For this review, take the finished solid that the model builds, in its own axes (mm). Face numbers are marked on the shaded views. Coordinates: 2 decimals unless noted, no trailing zeros. Order: outer loops, then holes, each group sorted by start corner. A loop starts at its lowest first (then second) coordinate and runs counter-clockwise, first axis right, second up. Notation, with made-up numbers: (-14.5, 51) -> (23.5, 51) arc R13 ccw to (23.5, 70) -> close; hole circle Ø9 at (-21, 27.5). An arc over 180 degrees is marked (long way). Answer as a JSON object with one key per item and string values. Group by question number.
1) For pin 1 (1 mm diameter, centred on x = -3, z = -14.5, fed in from -Y); pin 2 (3 mm diameter, centred on x = -4, z = -4, fed in from +Y); pin 3 (1 mm diameter, centred on x = -7, y = 4, fed in from -Z), all flat-tipped, find the tip position at first contact; note any pin that passes through.
2) Add section C-C, the plane z = -4.5. Write out the cut boundary in (x, y).
3) Draft analysis for pull direction Z (two halves, no side actions). For the marked faces 1, 2 and 3, state which applies: +Z half, -Z half, draft (parallel to the pull), parting line (faces both ways), or undercut.
4) Add section D-D, the plane x = -7. Write out the cut boundary in (y, z).
5) Add section A-A, the plane x = -4.5. Write out the cut boundary in (y, z).
6) Add section B-B, the plane y = 1.25. Count the separate pieces of the cut face and the enclosed holes in it, then the cut area to 3 significant figures.
7) Wall thickness on L1, parallel to Z at x = -4, y = 1.7; L2, parallel to X at y = 3.95, z = -4; L3, parallel to Z at x = -5.75, y = 3.4: over which ranges is each line inside the solid? List them lowest first.
Autodesk Inventor part; units mm, degrees
ref_plane "YZ Plane" through (0, 0, 0) normal (1, 0, 0) x (0, 1, 0)
ref_plane "XZ Plane" through (0, 0, 0) normal (0, 1, 0) x (-1, 0, 0)
ref_plane "XY Plane" through (0, 0, 0) normal (0, 0, 1) x (1, 0, 0)
sketch "Sketch1" plane through (0, 0, 0) normal (0, 1, 0) x (-1, 0, 0)
  line L0 (0, 0) -> (8, 0)
  line L1 (8, 0) -> (8, -45)
  line L2 (8, -45) -> (0, -45)
  line L3 (0, -45) -> (0, 0)
  line L4 (8, 0) -> (4, 0)
  line L5 (4, 0) -> (4, -4)
  circle A0 centre (4, -4) radius 2
  line L6 (8, -45) -> (4, -45)
  line L7 (4, -45) -> (4, -41)
  circle A1 centre (4, -41) radius 2
  dimension "d0" = 8
  dimension "d1" = 45
  dimension "d2" = 4
  dimension "d3" = 4
  dimension "d4" = 4
  dimension "d5" = 4
  dimension "d6" = 4
  dimension "d7" = 4
extrude "Extrusion1" add sketch "Sketch1" along normal blind 5
fillet "Fillet1" radius 4 4 edges at (0, 2.5, 0) (-8, 2.5, 0) (-8, 2.5, -45) (0, 2.5, -45)
properties part number "Bar"
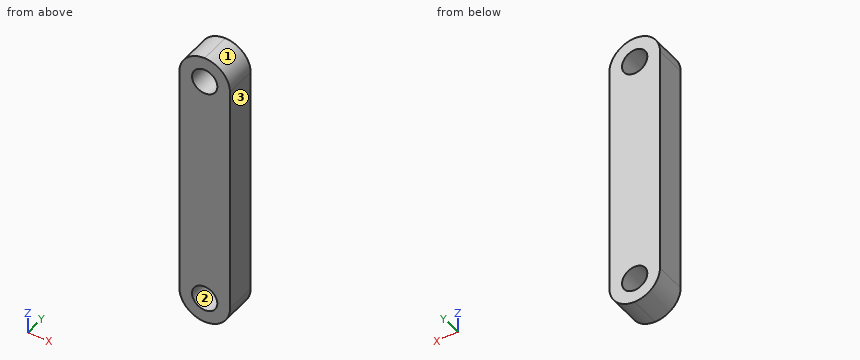
Output values:
{
 "1": {"pin 1": "stops at y = 0", "pin 2": "passes through", "pin 3": "stops at z = -44.12"},
 "2": {"outline": "(-8, 0) -> (-5.94, 0) -> (-5.94, 5) -> (-8, 5) -> close; (-2.06, 0) -> (0, 0) -> (0, 5) -> (-2.06, 5) -> close"},
 "3": {"face 1": "+Z half", "face 2": "undercut", "face 3": "draft"},
 "4": {"outline": "(0, -43.65) -> (5, -43.65) -> (5, -1.35) -> (0, -1.35) -> close"},
 "5": {"outline": "(0, -44.97) -> (5, -44.97) -> (5, -42.94) -> (0, -42.94) -> close; (0, -39.06) -> (5, -39.06) -> (5, -5.94) -> (0, -5.94) -> close; (0, -2.06) -> (5, -2.06) -> (5, -0.03) -> (0, -0.03) -> close"},
 "6": {"separate pieces": "1", "enclosed holes": "2", "area": "321 mm²"},
 "7": {"L1": "z = -45 to -43, -39 to -6, -2 to 0", "L2": "x = -8 to -6, -2 to 0", "L3": "z = -44.6 to -41.97, -40.03 to -4.97, -3.03 to -0.4"}
}
